The listing builds one solid part. Answer for the finished solid, in the listing's coordinates (mm). A direction names the side the tool comes from. Round coordinates to 2 decimals unless told otherwise and drop trailing zeros. Loops run counter-clockwise (first coordinate to the right, second up) from the corner with the lowest first, then second, coordinate; pieces in that order, holes last. Notation, with made-up numbers: (18.5, -25.5) -> (55.5, -25.5) arc R30 cw to (55.5, 13.5) -> close; hole circle Ø3 at (50.5, 1.25). An arc over 180 degrees is marked (long way). Use a Markdown table: item, result. Add a question column.
Q1. Section D-D on x = -13.5 is taken. Give the vertices of the cut face in (y, z), then the cut area to 3 significant figures.
Q2. Section A-A on x = 0 is taken. Give the vertices of the cut face in (y, z), then the cut area to 3 significant figures.
Q3. Section B-B on y = -45.72 is taken. Give the vertices of the cut face in (x, z).
Q4. Which of the six approach directions +Z, -Z, +X, -X, +Y, -Y give full straight-line access (tool end or side, diameter ignored) to faces 5 (the flat face through (-7, -20.828, 3)), 6 (the cylindrical face through (-28.976, 4.558, 3.131)), 7 (the flat face through (10, 19.62, 3.13))?
Q5. Given pin 1 Ø1.9 at (y, z) = (-40.5, 3.5) entering from +X; pin 2 Ø1.5 at (x, z) = (-13.5, 5.5) entering from +Y, each flat-ended and moving along its own axis, determine where each tip first touches the part or whether it passes through.
Q6. For a pull along Y with two mould halves and no side action, classify faces 1 (the flat face through (-30, -59.69, 3)), 2 (the cylindrical face through (-1.72, -7.75, 3.13)), 3 (the cylindrical face through (-13.31, 1.89, 3.13)), 4 (the flat face through (21.59, 12, 3)) as released by +Y, released by -Y, zero draft, split by the parting line, or undercut.
Q7. Consider line 1 (Y direction, x = 0, z = 4.25); line 2 (Y direction, x = 6.5, z = 2); line 3 (X direction, y = -34, z = 3.25). Determine where each line is inside the solid, lowest interval first.
Q8. Section C-C on z = 3.75 is taken. Give the vertices of the cut face in (x, y) (1 decimal), then the cut area to 3 significant figures.
from build123d import *

# Parameters (mm, degrees)
SKETCH1_R           = 3.048
SKETCH1_R_2         = 7.9375
BOSS_EXTRUDE1_DEPTH = 6.35


with BuildPart() as part:
    # Sketch1 → Boss-Extrude1 (new body)
    with BuildSketch(Plane.XY):
        with BuildLine():
            Line((21.59, 0), (21.59, 25.042396902))
            ThreePointArc((21.59, 25.042396902), (21.218025612, 25.940422514), (20.32, 26.312396902))
            Line((20.32, 26.312396902), (15.384027181, 26.312396902))
            Line((15.384027181, 26.312396902), (4.464894623, 12.734941429))
            ThreePointArc((4.464894623, 12.734941429), (3.875986132, 12.325731507), (3.159297438, 12.300765818))
            ThreePointArc((3.159297438, 12.300765818), (-6.605300924, 10.84711942), (-12.378605801, 2.839034768))
            ThreePointArc((-12.378605801, 2.839034768), (-13.326403154, 1.886506555), (-14.59892418, 2.318154625))
            Line((-14.59892418, 2.318154625), (-34.253888671, 26.312396902))
            Line((-34.253888671, 26.312396902), (-39.107436935, 26.312396902))
            ThreePointArc((-39.107436935, 26.312396902), (-40.005462547, 25.940422514), (-40.377436935, 25.042396902))
            Line((-40.377436935, 25.042396902), (-40.377436935, -58.42))
            ThreePointArc((-40.377436935, -58.42), (-40.005462547, -59.318025612), (-39.107436935, -59.69))
            Line((-39.107436935, -59.69), (-20.319056935, -59.69))
            Line((-20.319056935, -59.69), (-20.319056935, -20.828))
            Line((-20.319056935, -20.828), (5.685289439, -20.828))
            ThreePointArc((5.685289439, -20.828), (17.159159347, -13.103104613), (21.59, 0))
        make_face()
        with Locations((-30.382536935, 7.262396902)):
            Circle(SKETCH1_R, mode=Mode.SUBTRACT)
        Circle(SKETCH1_R_2, mode=Mode.SUBTRACT)
        with Locations((-30.382536935, -45.72)):
            Circle(SKETCH1_R, mode=Mode.SUBTRACT)
    extrude(amount=BOSS_EXTRUDE1_DEPTH)


solid = part.part
Checked values:
| question | item | result |
|---|---|---|
| 1 | outline | (-20.83, 0) -> (1.86, 0) -> (1.86, 6.35) -> (-20.83, 6.35) -> close |
| 1 | area | 144 mm2 |
| 2 | outline | (-20.83, 0) -> (-7.94, 0) -> (-7.94, 6.35) -> (-20.83, 6.35) -> close; (7.94, 0) -> (12.7, 0) -> (12.7, 6.35) -> (7.94, 6.35) -> close |
| 2 | area | 112 mm2 |
| 3 | outline | (-40.38, 0) -> (-33.43, 0) -> (-33.43, 6.35) -> (-40.38, 6.35) -> close; (-27.33, 0) -> (-20.32, 0) -> (-20.32, 6.35) -> (-27.33, 6.35) -> close |
| 4 | face 5 | +Z, -Z, +X, -Y |
| 4 | face 6 | +Z, -Z |
| 4 | face 7 | +Z, -Z, +Y |
| 5 | pin 1 | stops at x = -20.32 |
| 5 | pin 2 | stops at y = 2.19 |
| 6 | face 1 | released by -Y |
| 6 | face 2 | undercut |
| 6 | face 3 | released by +Y |
| 6 | face 4 | zero draft |
| 7 | line 1 | y = -20.83 to -7.94, 7.94 to 12.7 |
| 7 | line 2 | y = -20.59 to -4.56, 4.56 to 15.27 |
| 7 | line 3 | x = -40.38 to -20.32 |
| 8 | outline | (-40.4, -58.4) arc R1.3 ccw to (-39.1, -59.7) -> (-20.3, -59.7) -> (-20.3, -20.8) -> (5.7, -20.8) arc R21.6 ccw to (21.6, 0) -> (21.6, 25) arc R1.3 ccw to (20.3, 26.3) -> (15.4, 26.3) -> (4.5, 12.7) arc R1.3 cw to (3.2, 12.3) arc R12.7 ccw to (-12.4, 2.8) arc R1.3 cw to (-14.6, 2.3) -> (-34.3, 26.3) -> (-39.1, 26.3) arc R1.3 ccw to (-40.4, 25) -> close; hole circle Ø6.1 at (-30.4, -45.7); hole circle Ø6.1 at (-30.4, 7.3); hole circle Ø15.9 at (0, 0) |
| 8 | area | 2,730 mm2 |
